Can you work these out from the model? Positions are in its coordinate system, mm. Face numbers are marked on the shaded views. A direction names the side the tool comes from. Coordinates: 2 decimals unless noted, no trailing zeros. Loops run counter-clockwise (first coordinate to the right, second up) from the corner with the lowest first, then second, coordinate; pieces in that order, holes last. Notation, with made-up numbers: (13, 23.25) - (46, 23.25) arc R26 cw to (46, 54.25) - close; hole circle Ø9 at (52, -12.75). An arc over 180 degrees is marked (long way). Put each result on its own line as item: value. Start each with the question number.
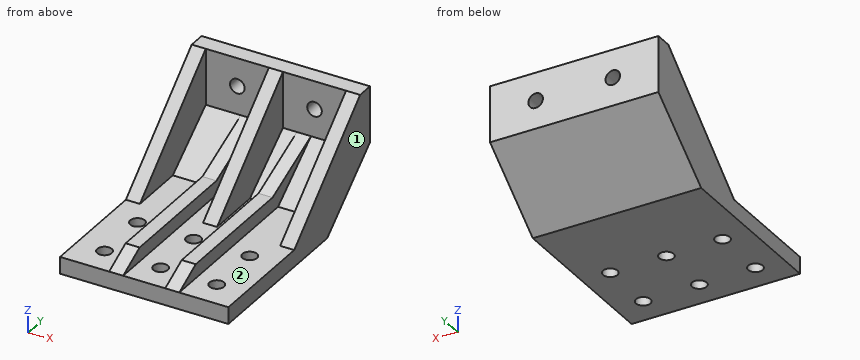
Autodesk Inventor part; units mm, degrees
ref_plane "Work Plane1" through (0, 0, 11) normal (0, 0, 1) x (1, 0, 0)
ref_plane "YZ Plane" through (0, 0, 0) normal (1, 0, 0) x (0, 1, 0)
ref_plane "XZ Plane" through (0, 0, 0) normal (0, 1, 0) x (-1, 0, 0)
sketch "Sketch1" plane through (0, 0, 0) normal (0, 0, 1) x (1, 0, 0)
  line L0 (0, 0) -> (-60, 0)
  line L1 (-60, 0) -> (-60, 60)
  line L2 (-60, 60) -> (0, 60)
  line L3 (0, 60) -> (0, 0)
  dimension "d0" = 60
  dimension "d1" = 60
extrude "Extrusion1" add sketch "Sketch1" along normal blind 6
sketch "Sketch2" plane through (0, 0, 6) normal (0, 0, 1) x (1, 0, 0)
  line L0 (0, 60) -> (-60, 60)
  line L1 (-60, 60) -> (-60, 0)
  line L2 (0, 60) -> (-60, 60)
  line L3 (-60, 60) -> (-60, 40)
  line L4 (-60, 40) -> (0, 40)
  line L5 (0, 40) -> (0, 60)
  line L6 (-60, 0) -> (0, 0) construction
  line L7 (-30, 0) -> (-30, 40) construction
  line L8 (-30, 20) -> (-30, 40) construction
  line L9 (-30, 20) -> (-30, 0) construction
  line L10 (-60, 30) -> (0, 30) construction
  line L11 (0, 0) -> (0, 60) construction
  line L12 (-60, 10) -> (0, 10) construction
  circle A0 centre (-50, 30) radius 2.6
  circle A1 centre (-30, 30) radius 2.6
  circle A2 centre (-10, 30) radius 2.6
  circle A3 centre (-50, 10) radius 2.6
  circle A4 centre (-30, 10) radius 2.6
  circle A5 centre (-10, 10) radius 2.6
  dimension "d4" = 20
  dimension "d5" = 5.2
  dimension "d6" = 5.2
  dimension "d7" = 5.2
  dimension "d8" = 5.2
  dimension "d9" = 5.2
  dimension "d10" = 5.2
  dimension "d11" = 20
  dimension "d12" = 20
  dimension "d13" = 20
  dimension "d14" = 20
  dimension "d15" = 20
extrude "Extrusion2" cut sketch "Sketch2" against normal up to next contours A0 | A1 | A2 | A3 | A4 | A5
sketch "Sketch3" plane through (0, 0, 0) normal (1, 0, 0) x (0, 0, -1)
  line L0 (0, 60) -> (0, 0) construction
  line L1 (0, 0) -> (0, 135.0487) construction
  line L2 (-21, 0) -> (-21, 135.0487) construction
  line L3 (-21, 86) -> (-41, 86)
  line L4 (-41, 86) -> (-41, 80)
  line L5 (-41, 80) -> (-21, 80)
  line L6 (-21, 80) -> (-21, 86)
  line L7 (0, 60) -> (-6, 60)
  line L8 (0, 60) -> (-6, 60)
  line L9 (-21, 86) -> (0, 60)
  line L10 (-6, 60) -> (-6, 0)
  line L11 (-6, 60) -> (-21, 80)
  dimension "d18" = 21
  dimension "d19" = 20
  dimension "d20" = 6
  dimension "d21" = 20
extrude "Extrusion3" add sketch "Sketch3" against normal up to surface (60 mm away)
sketch "Sketch4" plane through (0, 80, 41) normal (0, 0, 1) x (1, 0, 0)
  line L0 (0, 0) -> (-60, 0)
  line L1 (0, 0) -> (-5, 0)
  line L2 (-5, 0) -> (-5, -40)
  line L3 (-5, -40) -> (0, -40)
  line L4 (0, -40) -> (0, 0)
  circle A0 centre (-10, -50) radius 2.6
  line L5 (-32.5, 0) -> (-32.5, -40)
  line L6 (-27.5, 0) -> (-32.5, 0)
  line L7 (-27.5, -40) -> (-27.5, 0)
  line L8 (-32.5, -40) -> (-27.5, -40)
  line L9 (-60, 0) -> (-60, -40)
  line L10 (-55, 0) -> (-60, 0)
  line L11 (-55, -40) -> (-55, 0)
  line L12 (-60, -40) -> (-55, -40)
  point P0 (0, -80)
  dimension "d24" = 5
  dimension "d25" = 10
  dimension "d28" = 27.5
extrude "Extrusion4" add sketch "Sketch4" against normal up to next contours L4 L3 L2 L0 | L11 L12 L9 L0 | L7 L8 L5 L0
chamfer "Chamfer1" distance 40 distance2 35 1 edges at (-2.5, 40, 41) measured on face at (-30.8333, 84, 41)
chamfer "Chamfer2" distance 40 distance2 35 1 edges at (-30, 40, 41) measured on face at (-30.8333, 84, 41)
chamfer "Chamfer3" distance 40 distance2 35 1 edges at (-57.5, 40, 41) measured on face at (-30.8333, 84, 41)
sketch "Sketch5" plane through (-55, 80, 21) normal (0, -1, 0) x (1, 0, 0)
  line L0 (-5, 0) -> (-5, 20) construction
  line L1 (-5, 10) -> (55, 10) construction
  line L2 (55, -15) -> (55, 20) construction
  circle A0 centre (11.25, 10) radius 2.6
  circle A1 centre (38.75, 10) radius 2.6
  line L3 (0, 20) -> (0, 0)
  line L4 (27.5, 20) -> (27.5, 0)
  point P0 (55, -21)
  dimension "d44" = 5.2
  dimension "d45" = 5.2
  dimension "d46" = 11.25
  dimension "d47" = 11.25
extrude "Extrusion5" cut sketch "Sketch5" against normal up to next
ref_plane "Work Plane1" through (0, 0, 11) normal (0, 0, 1) x (1, 0, 0)
sketch "Sketch7" plane through (0, 0, 11) normal (0, 0, 1) x (1, 0, 0)
  line L0 (-60, 0) -> (0, 0)
  line L1 (-17.5, 0) -> (-22.5, 0)
  line L2 (-22.5, 0) -> (-22.5, 70)
  line L3 (-22.5, 70) -> (-17.5, 70)
  line L4 (-17.5, 70) -> (-17.5, 0)
  circle A0 centre (-10, 30) radius 2.6
  line L5 (-30, 0) -> (-30, 54.0913) construction
  line L6 (-42.5, 0) -> (-37.5, 0)
  line L7 (-37.5, 0) -> (-37.5, 70)
  line L8 (-37.5, 70) -> (-42.5, 70)
  line L9 (-42.5, 70) -> (-42.5, 0)
  dimension "d68" = 5
  dimension "d69" = 70
  dimension "d70" = 7.5
extrude "Extrusion7" add sketch "Sketch7" against normal up to next contours L9 L8 L7 L0 | L2 L3 L4 L0
chamfer "Chamfer8" distance 10 distance2 5 1 edges at (-20, 0, 11) measured on face at (-19.1667, 22.2222, 11)
chamfer "Chamfer9" distance 10 distance2 5 1 edges at (-40, 0, 11) measured on face at (-39.1667, 22.2222, 11)
chamfer "Chamfer10" distance 16.6667 distance2 10 1 edges at (-40, 66.6667, 11) measured on face at (-43.3333, 75.5556, 17.6667)
chamfer "Chamfer11" distance 16.6667 distance2 10 1 edges at (-20, 66.6667, 11) measured on face at (-16.6667, 75.5556, 17.6667)
equation "\"d6\" = d5"
equation "\"d7\" = d5"
equation "\"d8\" = d5"
equation "\"d9\" = d5"
equation "\"d10\" = d5"
equation "\"d47\" = d46"
properties part number "X Axis Drag Chain Support Mount"
Q1. On a 3-axis mill with a long thin cutter (end or side, diameter ignored), from which of +Z, -Z, +X, -X, +Y, -Y can I reach the whole of each face in a straight line? I mean the marked faces 1 and 2. Say none if no direction works.
Q2. Please list where these lines run through material, in increasing order: line 1 along X through (y, z) = (69, 26); line 2 along Y through (x, z) = (-10, 3); line 3 along Y through (x, z) = (-50, 1.3). Write a range as [from, to].
Q3. I want a section at D-D on z = 31. List the corners of the cut face in (x, y) for me.
Q4. I want a section at B-B on y = 19. List the corners of the cut face in (x, z) for me, and give its area (3 significant figures).
Q5. I want a section at C-C on x = -30. Count the separate pieces of the cut face and the enclosed holes in it, and give its area (3 significant figures).
Q6. Will these pins go through, and if not, where does the flat tip stop? pin 1 (4 mm diameter, centred on x = -40.5, y = 31, fed in from +Z); pin 2 (6 mm diameter, centred on x = -24.5, z = 15, fed in from +Y); pin 3 (7 mm diameter, centred on x = -43.75, z = 31, fed in from -Y).
Q7. I want a section at A-A on x = -43.75. List the corners of the cut face in (y, z) for me.
Calculated:
1. face 1: +Z, -Z, +X, +Y, -Y
1. face 2: +Z, -Y
2. line 1: [-60, -55], [-32.5, -27.5], [-5, 0]
2. line 2: [0, 7.4], [12.6, 27.4], [32.6, 63.71]
2. line 3: [0, 7.4], [12.6, 27.4], [32.6, 61.61]
3. outline: (-60, 68.57) - (-55, 68.57) - (-55, 80) - (-46.35, 80) - (-46.35, 86) - (-60, 86) - close; (-41.15, 80) - (-32.5, 80) - (-32.5, 68.57) - (-27.5, 68.57) - (-27.5, 80) - (-18.85, 80) - (-18.85, 86) - (-41.15, 86) - close; (-13.65, 80) - (-5, 80) - (-5, 68.57) - (0, 68.57) - (0, 86) - (-13.65, 86) - close
4. outline: (-60, 0) - (0, 0) - (0, 6) - (-17.5, 6) - (-17.5, 11) - (-22.5, 11) - (-22.5, 6) - (-37.5, 6) - (-37.5, 11) - (-42.5, 11) - (-42.5, 6) - (-60, 6) - close
4. area: 410 mm2
5. separate pieces: 3
5. enclosed holes: 0
5. area: 1,090 mm2
6. pin 1: z = 11
6. pin 2: y = 82.29
6. pin 3: y = 80
7. outline: (0, 0) - (60, 0) - (86, 21) - (86, 28.4) - (80, 28.4) - (80, 21) - (60, 6) - (0, 6) - close; (80, 33.6) - (86, 33.6) - (86, 41) - (80, 41) - close
